Read the model definition and answer for the solid it produces. Units are mm, in the model's axes. A direction names the side the tool comes from. Coordinates: 2 decimals unless noted, no trailing zeros. Write each loop counter-clockwise with the first axis right and the second up, starting at its lowest first coordinate (ties: lowest second). Pieces come first, ordered by that corner, then holes. Notation, with made-up numbers: (-30, 29.5) -> (-19, 29.5) arc R26 cw to (-19, 54.5) -> close; hole circle Ø4 at (55, -1.75). An arc over 180 degrees is marked (long way). Return JSON: item names as keys, results as strings.
from build123d import *

# Parameters (mm, degrees)
SKETCH_1_W           = 30.25
SKETCH_1_H           = 31
SKETCH_1_W_2         = 26.25
SKETCH_1_H_2         = 27
EXTRUDE_1_DEPTH      = 11.42
SKETCH_2_W           = 30.25
SKETCH_2_H           = 31
EXTRUDE_2_DEPTH      = 2.45
SKETCH_3_W           = 25.25
SKETCH_3_H           = 18.16
CUT_EXTRUDE_1_DEPTH  = 2.45
SKETCH_4_R           = 1.15
CUT_EXTRUDE_3_DEPTH  = 2.45
CUT_EXTRUDE_4_DEPTH  = 1.2
SKETCH_6_R           = 1.9
CUT_EXTRUDE_5_DEPTH  = 1.35
SKETCH_7_W           = 11
SKETCH_7_H           = 3.2
CUT_EXTRUDE_7_DEPTH  = 2.45
SKETCH_8_W           = 17
SKETCH_8_H           = 2
CUT_EXTRUDE_9_DEPTH  = 2.45
FILLET_1_R           = 1
SKETCH_12_W          = 6
SKETCH_12_H          = 6.9
CUT_EXTRUDE_10_DEPTH = 2
CUT_EXTRUDE_11_DEPTH = 2
SKETCH_15_W          = 9.5
SKETCH_15_H          = 8.4
CUT_EXTRUDE_12_DEPTH = 2
FILLET_2_R           = 0.5
FILLET_3_R           = 0.5
CUT_EXTRUDE_19_REACH = 36.644
SKETCH_17_W          = 26.25
SKETCH_17_H          = 2.1
SKETCH_18_W          = 3.8
SKETCH_18_H          = 2
CUT_EXTRUDE_20_DEPTH = 1.35


with BuildPart() as part:
    # 草图1 → 凸台-拉伸1 (new body)
    with BuildSketch(Plane(origin=(0, 0, 0), x_dir=(1, 0, 0), z_dir=(0, 1, 0))):
        Rectangle(SKETCH_1_W, SKETCH_1_H)
        Rectangle(SKETCH_1_W_2, SKETCH_1_H_2, mode=Mode.SUBTRACT)
    extrude(amount=-EXTRUDE_1_DEPTH)

    # 草图2 → 凸台-拉伸2 (add)
    with BuildSketch(Plane(origin=(0, 0, 0), x_dir=(1, 0, 0), z_dir=(0, 1, 0))):
        Rectangle(SKETCH_2_W, SKETCH_2_H)
    extrude(amount=EXTRUDE_2_DEPTH)

    # 草图3 → 切除-拉伸1 (cut)
    with BuildSketch(Plane(origin=(0, 0, 0), x_dir=(1, 0, 0), z_dir=(0, 1, 0))):
        with Locations((0, 0.08)):
            Rectangle(SKETCH_3_W, SKETCH_3_H)
    extrude(amount=CUT_EXTRUDE_1_DEPTH, mode=Mode.SUBTRACT)

    # 草图4 → 切除-拉伸3 (cut)
    with BuildSketch(Plane(origin=(0, 0, 0), x_dir=(1, 0, 0), z_dir=(0, 1, 0))):
        with Locations(Location((-10.625, 11, 0), (0, 0, 270))):
            Circle(SKETCH_4_R)
        with Locations(Location((-10.625, -11, 0), (0, 0, 90))):
            Circle(SKETCH_4_R)
        with Locations(Location((10.625, 11, 0), (0, 0, 90))):
            Circle(SKETCH_4_R)
        with Locations(Location((10.625, -11, 0), (0, 0, 270))):
            Circle(SKETCH_4_R)
    extrude(amount=CUT_EXTRUDE_3_DEPTH, mode=Mode.SUBTRACT)

    # 草图5 → 切除-拉伸4 (cut)
    with BuildSketch(Plane(origin=(0, 0, 0), x_dir=(1, 0, 0), z_dir=(0, 1, 0))):
        Polygon((-9.441431948, 8.95), (-8.257863896, 11), (-9.441431948, 13.05), (-11.808568052, 13.05), (-12.992136104, 11), (-11.808568052, 8.95), align=None)
        Polygon((11.808568052, 8.95), (9.441431948, 8.95), (8.257863896, 11), (9.441431948, 13.05), (11.808568052, 13.05), (12.992136104, 11), align=None)
    extrude(amount=CUT_EXTRUDE_4_DEPTH, mode=Mode.SUBTRACT)

    # 草图6 → 切除-拉伸5 (cut)
    with BuildSketch(Plane(origin=(0, 2.45, 0), x_dir=(1, 0, 0), z_dir=(0, 1, 0))):
        with Locations(Location((-10.625, -11, 0), (0, 0, 270))):
            Circle(SKETCH_6_R)
        with Locations(Location((10.625, -11, 0), (0, 0, 270))):
            Circle(SKETCH_6_R)
    extrude(amount=-CUT_EXTRUDE_5_DEPTH, mode=Mode.SUBTRACT)

    # 草图7 → 切除-拉伸7 (cut)
    with BuildSketch(Plane(origin=(0, 0, 0), x_dir=(1, 0, 0), z_dir=(0, 1, 0))):
        with Locations((0, -10.6)):
            Rectangle(SKETCH_7_W, SKETCH_7_H)
    extrude(amount=CUT_EXTRUDE_7_DEPTH, mode=Mode.SUBTRACT)

    # 草图8 → 切除-拉伸9 (cut)
    with BuildSketch(Plane(origin=(0, 0, 0), x_dir=(1, 0, 0), z_dir=(0, 1, 0))):
        with Locations((0, 11.7)):
            Rectangle(SKETCH_8_W, SKETCH_8_H)
    extrude(amount=CUT_EXTRUDE_9_DEPTH, mode=Mode.SUBTRACT)

    # 圆角1
    fillet_1_edges = [part.edges().sort_by_distance(p)[0] for p in [
        (-15.125, -4.485, -15.5),
        (15.125, -4.485, -15.5),
        (15.125, -4.485, 15.5),
        (-15.125, -4.485, 15.5),
    ]]
    fillet(fillet_1_edges, radius=FILLET_1_R)

    # 草图12 → 切除-拉伸10 (cut)
    with BuildSketch(Plane.ZY.offset(-13.125)):
        with Locations((-10.5, -7.97)):
            Rectangle(SKETCH_12_W, SKETCH_12_H)
    extrude(amount=-CUT_EXTRUDE_10_DEPTH, mode=Mode.SUBTRACT)

    # 草图14 → 切除-拉伸11 (cut)
    with BuildSketch(Plane.ZY.offset(-13.125)):
        with BuildLine():
            Line((2.857, -11.42), (2.857, -5.2))
            ThreePointArc((2.857, -5.2), (0.157, -2.5), (-2.543, -5.2))
            Line((-2.543, -5.2), (-2.543, -11.42))
            Line((-2.543, -11.42), (2.857, -11.42))
        make_face()
    extrude(amount=-CUT_EXTRUDE_11_DEPTH, mode=Mode.SUBTRACT)

    # 草图15 → 切除-拉伸12 (cut)
    with BuildSketch(Plane(origin=(-13.125, 0, 0), x_dir=(0, 0, -1), z_dir=(1, 0, 0))):
        with Locations((-3.25, -7.22)):
            Rectangle(SKETCH_15_W, SKETCH_15_H)
    extrude(amount=-CUT_EXTRUDE_12_DEPTH, mode=Mode.SUBTRACT)

    # 圆角2
    fillet_2_edges = [part.edges().sort_by_distance(p)[0] for p in [
        (-14.125, -3.02, 8),
        (-14.125, -3.02, -1.5),
    ]]
    fillet(fillet_2_edges, radius=FILLET_2_R)

    # 圆角3
    fillet_3_edges = [part.edges().sort_by_distance(p)[0] for p in [
        (-5.5, 1.225, 12.2),
        (5.5, 1.225, 12.2),
        (5.5, 1.225, 9),
        (-5.5, 1.225, 9),
    ]]
    fillet(fillet_3_edges, radius=FILLET_3_R)

    # 草图17 → 切除-拉伸19 (cut, up to next)
    with BuildSketch(Plane.XY.offset(-13.5), mode=Mode.PRIVATE) as cut_extrude_19_sk1:
        with Locations((0, -10.37)):
            Rectangle(SKETCH_17_W, SKETCH_17_H)
    cut_extrude_19_tool1 = extrude(cut_extrude_19_sk1.sketch, amount=-CUT_EXTRUDE_19_REACH, mode=Mode.PRIVATE) & part.part
    add(cut_extrude_19_tool1.solids().sort_by_distance((0, -10.37, -13.5))[0], mode=Mode.SUBTRACT)

    # 草图18 → 切除-拉伸20 (cut)
    with BuildSketch(Plane(origin=(0, 2.45, 0), x_dir=(1, 0, 0), z_dir=(0, 1, 0))):
        with Locations((-10.625, -10)):
            Rectangle(SKETCH_18_W, SKETCH_18_H)
        with Locations((10.625, -10)):
            Rectangle(SKETCH_18_W, SKETCH_18_H)
    extrude(amount=-CUT_EXTRUDE_20_DEPTH, mode=Mode.SUBTRACT)


solid = part.part
1. Flat-ended cylindrical pins translate along their axes: pin 1 Ø12 at (x, z) = (-2.5, -9.5) entering from -Y; pin 2 Ø1.9 at (x, z) = (-10, -10.5) entering from -Y; pin 3 Ø3 at (x, z) = (9.5, -10) entering from -Y. Find the tip coordinate at first contact, or state that the pin passes through.
Taken from the geometry:
{"pin 1": "stops at y = -9.32", "pin 2": "stops at y = 1.2", "pin 3": "stops at y = 0"}
2. Consider L1, parallel to X at y = 0.55, z = 11 (3 decimals); L2, parallel to X at y = 2, z = -11 (3 decimals); L3, parallel to Z at x = -10.5, y = 0.25. Determine where each line is inside the solid, lowest interval first.
Taken from the geometry:
{"L1": "x = -15.125 to -11.775, -9.475 to -5.5, 5.5 to 9.475, 11.775 to 15.125", "L2": "x = -15.125 to -11.775, -9.475 to -8.5, 8.5 to 9.475, 11.775 to 15.125", "L3": "z = -15.5 to -13.05, 9 to 9.86, 12.14 to 15.5"}
3. The part is cut by section C-C (z = 3.5). Determine the outline of the cut face in (x, y) (3 decimals).
Taken from the geometry:
{"outline": "(-15.125, -3.02) -> (-13.125, -3.02) -> (-13.125, 0) -> (-12.625, 0) -> (-12.625, 2.45) -> (-15.125, 2.45) -> close; (12.625, 0) -> (13.125, 0) -> (13.125, -11.42) -> (15.125, -11.42) -> (15.125, 2.45) -> (12.625, 2.45) -> close"}
4. For a pull along Z with two mould halves and no side action, classify faces 1 (the face through (0, 2.45, -14)), 2 (the face through (0, -5, -15.5)), 3 (the face through (14, -8, 2.857)) as +Z half, -Z half, draft (parallel to the pull), parting line (faces both ways), or undercut.
Taken from the geometry:
{"face 1": "draft", "face 2": "-Z half", "face 3": "undercut"}
5. A tool of negligible diameter and unlimited length cuts with its end or side. For faces 4 (the face through (-8.6, 0.9, 9)), 5 (the face through (14, -8, -2.543)), 6 (the face through (13.125, -10, -14)), 7 (the face through (-12, 1.2, -11)), from which of +Z, -Z, +X, -X, +Y, -Y can it reach the whole face along a straight path? Write none if from no direction.
Taken from the geometry:
{"face 4": "+Y, -Y", "face 5": "+X, -Y", "face 6": "-Z, -Y", "face 7": "-Y"}
6. The part is cut by section B-B (x = 0.5). Determine the outline of the cut face in (y, z), then the cut area to 3 significant figures.
Taken from the geometry:
{"outline": "(-11.42, 13.5) -> (0, 13.5) -> (0, 12.2) -> (2.45, 12.2) -> (2.45, 15.5) -> (-11.42, 15.5) -> close; (-9.32, -15.5) -> (2.45, -15.5) -> (2.45, -12.7) -> (0, -12.7) -> (0, -13.5) -> (-9.32, -13.5) -> close; (0, -10.7) -> (2.45, -10.7) -> (2.45, -9.16) -> (0, -9.16) -> close", "area": "60.2 mm2"}
7. The part is cut by section A-A (y = -6). Determine the outline of the cut face in (x, z) (3 decimals).
Taken from the geometry:
{"outline": "(-15.125, -14.5) arc R1 ccw to (-14.125, -15.5) -> (14.125, -15.5) arc R1 ccw to (15.125, -14.5) -> (15.125, -13.5) -> (-13.125, -13.5) -> (-13.125, -1.5) -> (-15.125, -1.5) -> close; (-15.125, 8) -> (-13.125, 8) -> (-13.125, 13.5) -> (13.125, 13.5) -> (13.125, 2.857) -> (15.125, 2.857) -> (15.125, 14.5) arc R1 ccw to (14.125, 15.5) -> (-14.125, 15.5) arc R1 ccw to (-15.125, 14.5) -> close; (13.125, -7.5) -> (15.125, -7.5) -> (15.125, -2.543) -> (13.125, -2.543) -> close"}
